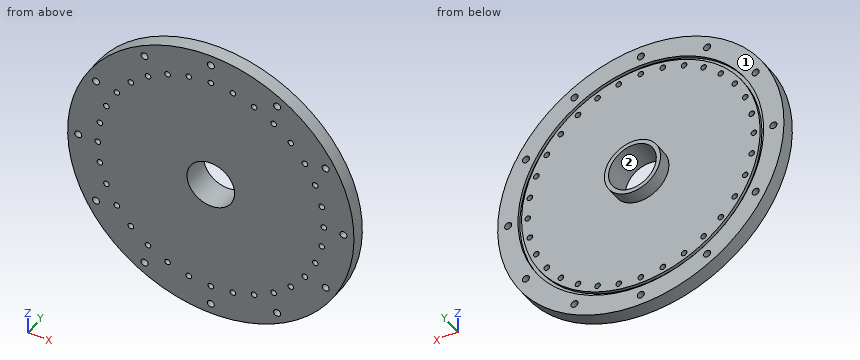
```python
from build123d import *

# Parameters (mm, degrees)
SKETCH1_R                  = 129.54
SKETCH1_R_2                = 21.59
SKETCH1_R_3                = 3.175
BOSS_EXTRUDE1_DEPTH        = 12.7
SKETCH2_R                  = 111.125
SKETCH2_R_2                = 107.95
CUT_EXTRUDE1_DEPTH         = 2.794
F_1_4_0_2_DIAMETER_HOLE1_D = 5.08
SKETCH5_R                  = 25.4
SKETCH5_R_2                = 21.59
BOSS_EXTRUDE2_DEPTH        = 12.7


with BuildPart() as part:
    # Sketch1 → Boss-Extrude1 (new body)
    with BuildSketch(Plane(origin=(0, 0, 0), x_dir=(1, 0, 0), z_dir=(0, 1, 0))):
        with Locations(Location((0, 0, 0), (0, 0, 270))):
            Circle(SKETCH1_R)
        with Locations(Location((0, 0, 0), (0, 0, 270))):
            Circle(SKETCH1_R_2, mode=Mode.SUBTRACT)
        with Locations(Location((0, 120.015, 0), (0, 0, 270))):
            Circle(SKETCH1_R_3, mode=Mode.SUBTRACT)
        with Locations(Location((60.0075, 103.936038835, 0), (0, 0, 270))):
            Circle(SKETCH1_R_3, mode=Mode.SUBTRACT)
        with Locations(Location((103.936038835, 60.0075, 0), (0, 0, 270))):
            Circle(SKETCH1_R_3, mode=Mode.SUBTRACT)
        with Locations(Location((120.015, 0, 0), (0, 0, 270))):
            Circle(SKETCH1_R_3, mode=Mode.SUBTRACT)
        with Locations(Location((103.936038835, -60.0075, 0), (0, 0, 270))):
            Circle(SKETCH1_R_3, mode=Mode.SUBTRACT)
        with Locations(Location((60.0075, -103.936038835, 0), (0, 0, 270))):
            Circle(SKETCH1_R_3, mode=Mode.SUBTRACT)
        with Locations(Location((0, -120.015, 0), (0, 0, 270))):
            Circle(SKETCH1_R_3, mode=Mode.SUBTRACT)
        with Locations(Location((-60.0075, -103.936038835, 0), (0, 0, 270))):
            Circle(SKETCH1_R_3, mode=Mode.SUBTRACT)
        with Locations(Location((-103.936038835, -60.0075, 0), (0, 0, 270))):
            Circle(SKETCH1_R_3, mode=Mode.SUBTRACT)
        with Locations(Location((-120.015, 0, 0), (0, 0, 270))):
            Circle(SKETCH1_R_3, mode=Mode.SUBTRACT)
        with Locations(Location((-103.936038835, 60.0075, 0), (0, 0, 270))):
            Circle(SKETCH1_R_3, mode=Mode.SUBTRACT)
        with Locations(Location((-60.0075, 103.936038835, 0), (0, 0, 270))):
            Circle(SKETCH1_R_3, mode=Mode.SUBTRACT)
    extrude(amount=BOSS_EXTRUDE1_DEPTH)

    # Sketch2 → Cut-Extrude1 (cut)
    with BuildSketch(Plane(origin=(0, 12.7, 0), x_dir=(1, 0, 0), z_dir=(0, 1, 0))):
        with Locations(Location((0, 0, 0), (0, 0, 270))):
            Circle(SKETCH2_R)
        with Locations(Location((0, 0, 0), (0, 0, 270))):
            Circle(SKETCH2_R_2, mode=Mode.SUBTRACT)
    extrude(amount=-CUT_EXTRUDE1_DEPTH, mode=Mode.SUBTRACT)

    # 1/4 (0.2) Diameter Hole1 (through all)
    with Locations(Plane(origin=(19.959924954, 12.7, -100.34531898), x_dir=(0, 0, 1), z_dir=(0, 1, 0))):
        with Locations((0, 0), (5.822095353, 19.192876231), (15.276665182, 36.881132271), (28.000375669, 52.385018357), (43.504261755, 65.108728844), (61.192517795, 74.563298673), (80.385394026, 80.385394026), (100.34531898, 82.351275046), (120.305243934, 80.385394026), (139.498120165, 74.563298673), (157.186376204, 65.108728844), (172.690262291, 52.385018357), (185.413972778, 36.881132271), (194.868542607, 19.192876231), (200.69063796, 0), (202.65651898, -19.959924954), (200.69063796, -39.919849908), (194.868542607, -59.112726139), (185.413972778, -76.800982178), (172.690262291, -92.304868265), (157.186376205, -105.028578752), (139.498120165, -114.483148581), (120.305243934, -120.305243934), (100.34531898, -122.271124954), (80.385394026, -120.305243934), (61.192517795, -114.483148581), (43.504261756, -105.028578752), (28.000375669, -92.304868265), (15.276665182, -76.800982179), (5.822095353, -59.112726139), (0, -39.919849908), (-1.96588102, -19.959924954)):
            Hole(F_1_4_0_2_DIAMETER_HOLE1_D / 2)

    # Sketch5 → Boss-Extrude2 (add)
    with BuildSketch(Plane(origin=(0, 12.7, 0), x_dir=(1, 0, 0), z_dir=(0, 1, 0))):
        with Locations(Location((0, 0, 0), (0, 0, 270))):
            Circle(SKETCH5_R)
        with Locations(Location((0, 0, 0), (0, 0, 270))):
            Circle(SKETCH5_R_2, mode=Mode.SUBTRACT)
    extrude(amount=BOSS_EXTRUDE2_DEPTH)


solid = part.part
```
Input: part model. Units: mm. Frame: model coordinates. Face numbers are marked on the shaded views. Round coordinates to 2 decimals unless told otherwise and drop trailing zeros. Loops run counter-clockwise (first coordinate to the right, second up) from the corner with the lowest first, then second, coordinate; pieces in that order, holes last. Notation, with made-up numbers: (7.5, 69.5) -> (31.5, 69.5) arc R36 ccw to (31.5, 103.5) -> close; hole circle Ø4 at (4, 28). An arc over 180 degrees is marked (long way). Use one line per item in the form item = value. Start each with the question number.
Item 1: Section query B-B on y = 16.25. Return the cut outline in (x, z), then the cut area to 3 significant figures.
Item 2: Section query A-A on z = 12. Return the cut outline in (x, y), then the cut area to 3 significant figures.
Item 3: Section query C-C on x = -46. Return the cut outline in (y, z), then the cut area to 3 significant figures.
Item 4: Material intervals for L1, parallel to X at y = 4.75, z = -73.5; L2, parallel to Y at x = 50.5, z = -114; L3, parallel to Z at x = -46, y = 12.5, sorted ascending. Write a range as from..to.
Item 5: Mould query, pull axis X, two halves, no side actions, for the marked faces 1 and 2. Classes: pulls with the +X half, pulls with the -X half, needs draft (parallel to the pull), parting line crosses it, or undercut.
Item 6: Contact query for flat-ended pins moving along their axis: pin 1 Ø5 at (y, z) = (9, 43) entering from +X; pin 2 Ø6 at (y, z) = (10, 49.5) entering from +X; pin 3 Ø12 at (y, z) = (21, 26) entering from +X; pin 4 Ø4.5 at (x, z) = (94.52, -39.15) entering from +Y. Output: stop coordinate, or through.
Ans:
q1.outline = circle Ø50.8 at (0, 0); hole circle Ø43.18 at (0, 0)
q1.area = 562 mm^2
q2.outline = (-128.98, 0) -> (-17.95, 0) -> (-17.95, 25.4) -> (-22.39, 25.4) -> (-22.39, 12.7) -> (-107.28, 12.7) -> (-107.28, 9.91) -> (-110.48, 9.91) -> (-110.48, 12.7) -> (-128.98, 12.7) -> close; (17.95, 0) -> (128.98, 0) -> (128.98, 12.7) -> (110.48, 12.7) -> (110.48, 9.91) -> (107.28, 9.91) -> (107.28, 12.7) -> (22.39, 12.7) -> (22.39, 25.4) -> (17.95, 25.4) -> close
q2.area = 2,920 mm^2
q3.outline = (0, -121.1) -> (12.7, -121.1) -> (12.7, -101.16) -> (9.91, -101.16) -> (9.91, -97.66) -> (12.7, -97.66) -> (12.7, 97.66) -> (9.91, 97.66) -> (9.91, 101.16) -> (12.7, 101.16) -> (12.7, 121.1) -> (0, 121.1) -> close
q3.area = 3,060 mm^2
q4.L1 = -106.67..-74.61, -70.08..70.08, 74.61..106.67
q4.L2 = 0..12.7
q4.L3 = -121.1..-101.16, -97.66..97.66, 101.16..121.1
q5.face_1 = needs draft
q5.face_2 = undercut
q6.pin_1 = 123.05
q6.pin_2 = 120.91
q6.pin_3 = 15.66
q6.pin_4 = through
